Geometry: final body of the model. Coordinates: model frame, mm. Face numbers are marked on the shaded views. A direction names the side the tool comes from. Give positions to 0.01 mm unless a question says otherwise; leave off trailing zeros. Order: outer loops, then holes, each group sorted by start corner. A loop starts at its lowest first (then second) coordinate and runs counter-clockwise, first axis right, second up. Notation, with made-up numbers: (49.25, -20.75) -> (68.25, -20.75) arc R17 cw to (68.25, -16.75) -> close; hole circle Ø4 at (50.5, 31). An arc over 180 degrees is marked (long way). Answer in a Markdown table with one row per item. Add a question column.
Q1. Set-up query: the marked faces 1 and 2. Return all of +Z, -Z, +X, -X, +Y, -Y with unobstructed straight access to the full face (end or side cutting, diameter ignored); none if empty.
Q2. Cut plane C-C on z = 0. Return the cut outline in (x, y), and give its area (3 significant figures).
Q3. Cut plane B-B on x = 38.5. Return the cut outline in (y, z), and give its area (3 significant figures).
Q4. Pull-direction query (Y, two-part tool) for the marked faces 3, 4 and 5; classes: +Y half, -Y half, draft (parallel to the pull), parting line (faces both ways), or undercut.
Q5. Line query: line 1 along Z through (x, y) = (37, 9.5); line 2 along X through (y, z) = (1.5, 3); line 3 along Z through (x, y) = (43, 1). Output: solid intervals per line, ascending. Write a range as from..to.
Q6. Cut plane D-D on x = 19. Return the cut outline in (y, z).
Q7. Cut plane A-A on y = 0. Return the cut outline in (x, z), and give its area (3 significant figures).
Q8. Contact query for flat-ended pins moving along their axis: P1, Ø6, axis at x = 28.5, z = -8.5, coming from the +Y side; P2, Ø2, axis at y = 0.5, z = 0.5, coming from the +X side; P3, Ø10, axis at x = 25, y = 13, coming from the +Z side. Output: stop coordinate, or through.
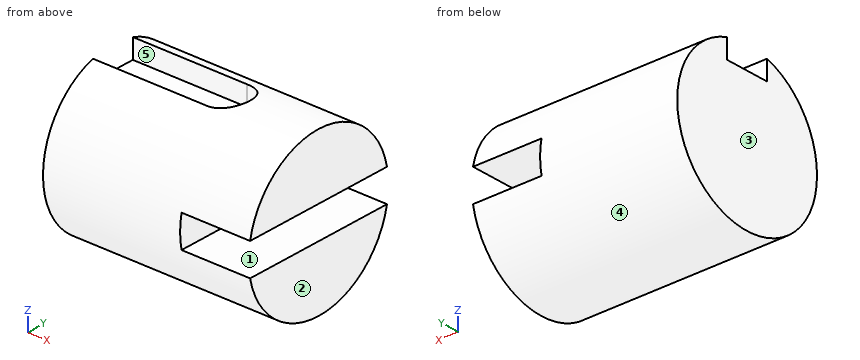
from build123d import *

# Parameters (mm, degrees)
F0_R     = 17.5
F1_DEPTH = 45
F3_DEPTH = 15
F6_DEPTH = 10


with BuildPart() as f1:
    # F0 (on Right) → F1 (new body)
    with BuildSketch(Plane.YZ):
        Circle(F0_R)
    extrude(amount=F1_DEPTH)

    # F2 (on face) → F3 (cut)
    with BuildSketch(Plane.YZ.offset(45)):
        with BuildLine():
            Line((17.1464281995, 3.5), (-17.1464281995, 3.5))
            ThreePointArc((-17.1464281995, 3.5), (-17.5, 0), (-17.1464281995, -3.5))
            Line((-17.1464281995, -3.5), (17.1464281995, -3.5))
            ThreePointArc((17.1464281995, -3.5), (17.4113826776, -1.7589068351), (17.5, 0))
            ThreePointArc((17.5, 0), (17.4113826776, 1.7589068351), (17.1464281995, 3.5))
        make_face()
    extrude(amount=-F3_DEPTH, mode=Mode.SUBTRACT)

    # F5 (on offset) → F6 (cut)
    with BuildSketch(Plane.XY.offset(12.5)):
        with BuildLine():
            Line((25, 5), (0, 5))
            Line((0, 5), (0, -5))
            Line((0, -5), (25, -5))
            ThreePointArc((25, -5), (30, 0), (25, 5))
        make_face()
    extrude(amount=F6_DEPTH, mode=Mode.SUBTRACT)


solid = f1.part
Completed:
| question | item | result |
|---|---|---|
| 1 | face 1 | +X, +Y, -Y |
| 1 | face 2 | +Z, -Z, +X, +Y, -Y |
| 2 | outline | (0, -17.5) -> (30, -17.5) -> (30, 17.5) -> (0, 17.5) -> close |
| 2 | area | 1,050 mm² |
| 3 | outline | (-17.15, -3.5) arc R17.5 ccw to (17.15, -3.5) -> close; (-17.15, 3.5) -> (17.15, 3.5) arc R17.5 ccw to start |
| 3 | area | 719 mm² |
| 4 | face 3 | draft |
| 4 | face 4 | parting line |
| 4 | face 5 | undercut |
| 5 | line 1 | z = -14.7..-3.5, 3.5..14.7 |
| 5 | line 2 | x = 0..30 |
| 5 | line 3 | z = -17.47..-3.5, 3.5..17.47 |
| 6 | outline | (-5, 12.5) -> (-5, 16.77) arc R17.5 ccw (long way) to (5, 16.77) -> (5, 12.5) -> close |
| 7 | outline | (0, -17.5) -> (45, -17.5) -> (45, -3.5) -> (30, -3.5) -> (30, 3.5) -> (45, 3.5) -> (45, 17.5) -> (30, 17.5) -> (30, 12.5) -> (0, 12.5) -> close |
| 7 | area | 1,320 mm² |
| 8 | P1 | stops at y = 16.61 |
| 8 | P2 | stops at x = 30 |
| 8 | P3 | stops at z = 15.56 |
